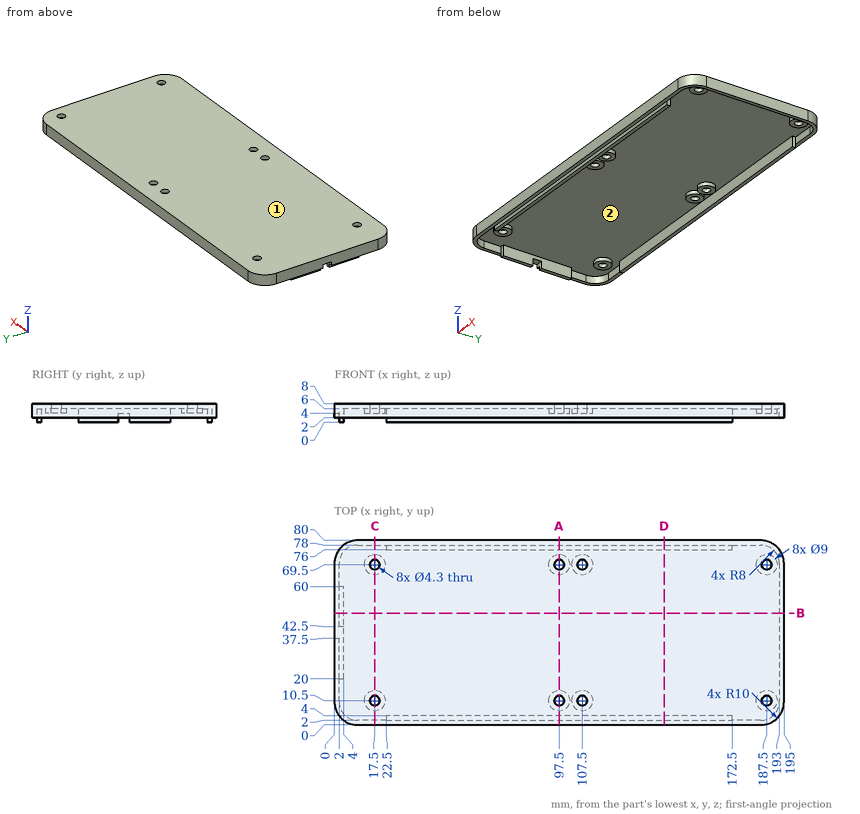
Drawing for the job (mm, zero at the part's lowest x, y, z). Give positions to 0.01 mm unless a question says otherwise; leave off trailing zeros. Order: outer loops, then holes, each group sorted by start corner. A loop starts at its lowest first (then second) coordinate and runs counter-clockwise, first axis right, second up. Notation, with made-up numbers: M -5.75,41 L 27.25,41 A22 cw 27.25,69 Z; hole C -32,59 d1. An arc over 180 degrees is marked long. Put each result on its own line as item: value. Start each with the question number.
(1) Mould opens along Y. For the marked faces 1 and 2 say: +Y half, -Y half, draft (parallel to the pull), parting line (faces both ways), or undercut.
(2) Flat gauge pins, fed straight in: pin 1 Ø5.5 at (x, y) = (17.5, 69.5) entering from +Z; pin 2 Ø0.6 at (y, z) = (3, 2) entering from -X; pin 3 Ø10 at (x, y) = (188.5, 9.5) entering from -Z; pin 4 Ø5 at (x, y) = (17.5, 10.5) entering from -Z. Where does each tip first touch, or does it go through?
(3) Saw through at C-C, the plane x = 17.5. Write the cut outline in (y, z), then the cut area to 3 significant figures.
(4) Drill centre lines: line 1 along Y through (x, z) = (107.5, 6.4); line 2 along Y through (x, z) = (17.5, 4.95); line 3 along X through (y, z) = (69.5, 6.5). Where is each one in solid material? Low to high.
(5) Saw through at B-B, the plane y = 48.5. Write the cut outline in (x, z), then the cut area to 3 significant figures.
(6) Saw through at A-A, the plane x = 97.5. Write the cut outline in (y, z).
(7) Saw through at D-D, the plane x = 143. Write the cut outline in (y, z), then the cut area to 3 significant figures.
Check result:
1. face 1: draft
1. face 2: undercut
2. pin 1: stops at z = 8
2. pin 2: stops at x = 2.58
2. pin 3: stops at z = 2
2. pin 4: stops at z = 4
3. outline: M 0,2 L 2,2 L 2,6 L 6,6 L 6,4 L 8.35,4 L 8.35,8 L 0,8 Z; M 12.65,4 L 15,4 L 15,6 L 65,6 L 65,4 L 67.35,4 L 67.35,8 L 12.65,8 Z; M 71.65,4 L 74,4 L 74,6 L 78,6 L 78,2 L 80,2 L 80,8 L 71.65,8 Z
3. area: 178 mm2
4. line 1: y = 0 to 8.35, 12.65 to 67.35, 71.65 to 80
4. line 2: y = 0 to 2, 6 to 8.35, 12.65 to 15, 65 to 67.35, 71.65 to 74, 78 to 80
4. line 3: x = 0 to 15.35, 19.65 to 95.35, 99.65 to 105.35, 109.65 to 185.35, 189.65 to 195
5. outline: M 0,2 L 2,2 L 2,0 L 4,0 L 4,6 L 193,6 L 193,2 L 195,2 L 195,8 L 0,8 Z
5. area: 418 mm2
6. outline: M 0,2 L 2,2 L 2,0 L 4,0 L 4,6 L 6,6 L 6,4 L 8.35,4 L 8.35,8 L 0,8 Z; M 12.65,4 L 15,4 L 15,6 L 65,6 L 65,4 L 67.35,4 L 67.35,8 L 12.65,8 Z; M 71.65,4 L 74,4 L 74,6 L 76,6 L 76,0 L 78,0 L 78,2 L 80,2 L 80,8 L 71.65,8 Z
7. outline: M 0,2 L 2,2 L 2,0 L 4,0 L 4,6 L 76,6 L 76,0 L 78,0 L 78,2 L 80,2 L 80,8 L 0,8 Z
7. area: 200 mm2
